Geometry: final body of the model. Coordinates: model frame, mm. Face numbers are marked on the shaded views. A direction names the side the tool comes from. Give positions to 0.01 mm unless a question says otherwise; leave off trailing zeros. Order: outer loops, then holes, each group sorted by start corner. A loop starts at its lowest first (then second) coordinate and runs counter-clockwise, first axis right, second up. Notation, with made-up numbers: (-25.75, 48.25) - (18.25, 48.25) arc R16 cw to (18.25, 71.25) - close; hole circle Ø2 at (72, 62). An arc over 180 degrees is marked (long way). Use one line per item in the form item = value.
Autodesk Inventor part; units mm, degrees
ref_plane "YZ Plane" through (0, 0, 0) normal (1, 0, 0) x (0, 1, 0)
ref_plane "XZ Plane" through (0, 0, 0) normal (0, 1, 0) x (-1, 0, 0)
ref_plane "XY Plane" through (0, 0, 0) normal (0, 0, 1) x (1, 0, 0)
sketch "Sketch1" plane through (0, 0, 0) normal (0, 0, 1) x (1, 0, 0)
  line L0 (-43, -26) -> (43, -26)
  line L1 (43, -26) -> (43, -16)
  line L2 (28, 26) -> (-28, 26)
  line L3 (-43, -16) -> (-43, -26)
  line L4 (-28, 26) -> (-28, -16)
  line L5 (-28, -16) -> (-43, -16)
  line L6 (28, 26) -> (28, -16)
  line L7 (28, -16) -> (43, -16)
  circle A0 centre (0, 1) radius 22.5
  point P0 (0, 0)
  point P1 (35.5, -16)
  dimension "d4" = 52
  dimension "d5" = 42
  dimension "d6" = 56
  dimension "d7" = 86
  dimension "d8" = 10
  dimension "d9" = 27
  dimension "d10" = 45
extrude "Extrusion1" add sketch "Sketch1" along normal blind 15.875
sketch "Sketch2" plane through (0, 0, 15.875) normal (0, 0, 1) x (1, 0, 0)
  circle A0 centre (0, 1) radius 22.5
  point P0 (0, 0)
extrude "Extrusion2" add sketch "Sketch2" against normal blind 3.875
sketch "Sketch3" plane through (0, 1, 12) normal (0, 0, -1) x (-1, 0, 0)
  circle A0 centre (0, 0) radius 8
  point P0 (0, -1)
  dimension "d15" = 16
extrude "Extrusion3" cut sketch "Sketch3" against normal blind 3.875
properties part number "Dudukan PG45"
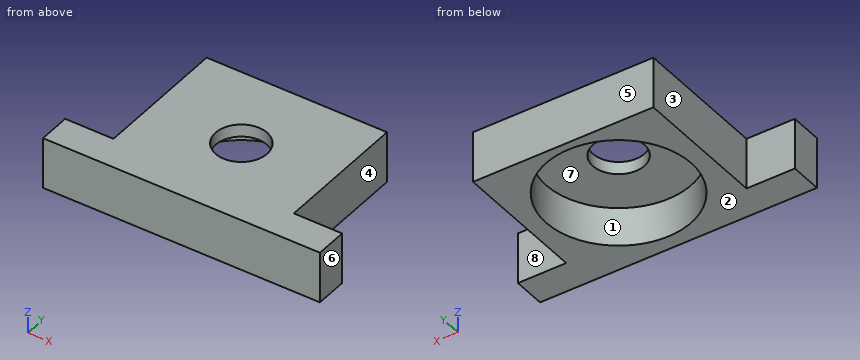
(1) Cut plane D-D on x = 32. Output: boundary loops of the cut face in (y, z) (3 decimals), plus the area to 3 significant figures.
Computed values:
outline = (-26, 0) - (-16, 0) - (-16, 15.875) - (-26, 15.875) - close
area = 159 mm²
(2) Ray query, line 1 along X through (y, z) = (0.5, 5.25); line 2 along Y through (x, z) = (0, 15.05); line 3 along Y through (x, z) = (0, 3.5). Return the intervals inside material, ascending.
Computed values:
line_1 = -28 to -22.49, 22.49 to 28
line_2 = -26 to -7, 9 to 26
line_3 = -26 to -21.5, 23.5 to 26
(3) Cut plane A-A on x = 0. Output: boundary loops of the cut face in (y, z) (3 decimals), plus the area to 4 significant figures.
Computed values:
outline = (-26, 0) - (-21.5, 0) - (-21.5, 12) - (-7, 12) - (-7, 15.875) - (-26, 15.875) - close; (9, 12) - (23.5, 12) - (23.5, 0) - (26, 0) - (26, 15.875) - (9, 15.875) - close
area = 223.5 mm²
(4) Contact query for flat-ended pins moving along their axis: pin 1 Ø4.5 at (x, z) = (39, 4) entering from +Y; pin 2 Ø8 at (y, z) = (4, 9.5) entering from -X; pin 3 Ø3 at (x, y) = (20, -5) entering from -Z. Output: stop coordinate, or through.
Computed values:
pin_1 = -16
pin_2 = -28
pin_3 = 12
(5) Pull-direction query (Y, two-part tool) for the marked faces 6, 7 and 8; classes: released by +Y, released by -Y, zero draft, split by the parting line, or undercut.
Computed values:
face_6 = zero draft
face_7 = undercut
face_8 = released by +Y
(6) Cut plane B-B on z = 8. Output: boundary loops of the cut face in (x, y).
Computed values:
outline = (-43, -26) - (43, -26) - (43, -16) - (28, -16) - (28, 26) - (-28, 26) - (-28, -16) - (-43, -16) - close; hole circle Ø45 at (0, 1)
(7) Cut plane C-C on y = 1. Output: boundary loops of the cut face in (x, z) (3 decimals), plus the area to 3 significant figures.
Computed values:
outline = (-28, 0) - (-22.5, 0) - (-22.5, 12) - (-8, 12) - (-8, 15.875) - (-28, 15.875) - close; (8, 12) - (22.5, 12) - (22.5, 0) - (28, 0) - (28, 15.875) - (8, 15.875) - close
area = 287 mm²
(8) Reachability of the marked faces 1, 2, 3, 4 and 5 from +Z, -Z, +X, -X, +Y, -Y: full face, straight path, thin tool, end or side. Return the list, or none.
Computed values:
face_1 = -Z
face_2 = -Z, +X, -X, +Y, -Y
face_3 = +Z, -Z, -X, +Y
face_4 = +Z, -Z, +X, +Y
face_5 = +Z, -Z, +X, -X, +Y
